from build123d import *

# Parameters (mm, degrees)
EXTRUDE_1_DEPTH     = 40
SKETCH_2_R          = 2.1
CUT_EXTRUDE_1_DEPTH = 3
SKETCH_3_R          = 11.1
SKETCH_3_R_2        = 1.6
CUT_EXTRUDE_2_DEPTH = 3
FILLET_1_R          = 3
FILLET_2_R          = 12
FILLET_3_R          = 1
FILLET_4_R          = 1


with BuildPart() as part:
    # 草图1 → 凸台-拉伸1 (new body)
    with BuildSketch(Plane.XY):
        Polygon((0, 3), (0, 0), (38.5, 0), (41.5, 0), (41.5, 3), (41.5, 42), (38.5, 42), (38.5, 3), align=None)
    extrude(amount=EXTRUDE_1_DEPTH)

    # 草图2 → 切除-拉伸1 (cut)
    with BuildSketch(Plane(origin=(41.5, 0, 0), x_dir=(0, 0, -1), z_dir=(1, 0, 0))):
        with Locations((-35, 34)):
            Circle(SKETCH_2_R)
        with Locations((-5, 34)):
            Circle(SKETCH_2_R)
        with Locations((-35, 9)):
            Circle(SKETCH_2_R)
        with Locations((-5, 9)):
            Circle(SKETCH_2_R)
    extrude(amount=-CUT_EXTRUDE_1_DEPTH, mode=Mode.SUBTRACT)

    # 草图3 → 切除-拉伸2 (cut)
    with BuildSketch(Plane.XZ):
        with Locations((18.5, 20)):
            Circle(SKETCH_3_R)
        with Locations((8.600505063, 29.899494937)):
            Circle(SKETCH_3_R_2)
        with Locations((28.399494937, 29.899494937)):
            Circle(SKETCH_3_R_2)
        with Locations((28.399494937, 10.100505063)):
            Circle(SKETCH_3_R_2)
        with Locations((8.600505063, 10.100505063)):
            Circle(SKETCH_3_R_2)
    extrude(amount=-CUT_EXTRUDE_2_DEPTH, mode=Mode.SUBTRACT)

    # 圆角1
    fillet_1_edges = [part.edges().sort_by_distance(p)[0] for p in [
        (41.5, 0, 20),
    ]]
    fillet(fillet_1_edges, radius=FILLET_1_R)

    # 圆角2
    fillet_2_edges = [part.edges().sort_by_distance(p)[0] for p in [
        (0, 1.5, 40),
        (0, 1.5, 0),
    ]]
    fillet(fillet_2_edges, radius=FILLET_2_R)

    # 圆角3
    fillet_3_edges = [part.edges().sort_by_distance(p)[0] for p in [
        (40, 42, 40),
        (40, 42, 0),
    ]]
    fillet(fillet_3_edges, radius=FILLET_3_R)

    # 圆角4
    fillet_4_edges = [part.edges().sort_by_distance(p)[0] for p in [
        (38.5, 3, 20),
    ]]
    fillet(fillet_4_edges, radius=FILLET_4_R)


solid = part.part
Part model, mm, in its own coordinate system. A direction names the side the tool comes from. Coordinates: 2 decimals unless noted, no trailing zeros. Order: outer loops, then holes, each group sorted by start corner. A loop starts at its lowest first (then second) coordinate and runs counter-clockwise, first axis right, second up. Notation, with made-up numbers: (39, -27) - (50, -27) arc R28 cw to (50, -9) - close; hole circle Ø8 at (58.25, 2). An arc over 180 degrees is marked (long way). Use CSV: the item, a comma, the result in double quotes.
Item 1: Probe probe 1 along Y at (x, z) = (40.5, 6); probe 2 along Y at (x, z) = (6.5, 26.5); probe 3 along X at (y, z) = (22, 27). List the from-to ranges inside material, lowest first.
Solved:
probe 1,"y = 0.76 to 7.15, 10.85 to 32.15, 35.85 to 42"
probe 2,"y = 0 to 3"
probe 3,"x = 38.5 to 41.5"
Item 2: Drop flat-ended pins along their axis: P1, Ø6.5, axis at y = 34, z = 5, coming from the +X side; P2, Ø12, axis at y = 31, z = 16, coming from the -X side; P3, Ø5, axis at x = 28.4, z = 10.1, coming from the +Y side. Give the stop position or say it passes through.
Solved:
P1,"stops at x = 41.5"
P2,"stops at x = 38.5"
P3,"stops at y = 3"
Item 3: Mould opens along X. For faces 3 (the face through (40.02, 31.95, 5.46)), 4 (the face through (40.6, 0.86, 20.28)), 5 (the face through (28.754, 1.479, 15.749)) say: +X half, -X half, draft (parallel to the pull), parting line (faces both ways), or undercut.
Solved:
face 3,"draft"
face 4,"+X half"
face 5,"undercut"
Item 4: Saw through at C-C on z = 20. Give the cut face in (x, y), and give its area (3 significant figures).
Solved:
outline,"(0, 0) - (7.4, 0) - (7.4, 3) - (0, 3) - close; (29.6, 0) - (38.5, 0) arc R3 ccw to (41.5, 3) - (41.5, 42) - (38.5, 42) - (38.5, 4) arc R1 cw to (37.5, 3) - (29.6, 3) - close"
area,"173 mm²"
Item 5: Saw through at A-A on y = 34. Give the cut face in (x, z).
Solved:
outline,"(38.5, 0) - (41.5, 0) - (41.5, 2.9) - (38.5, 2.9) - close; (38.5, 7.1) - (41.5, 7.1) - (41.5, 32.9) - (38.5, 32.9) - close; (38.5, 37.1) - (41.5, 37.1) - (41.5, 40) - (38.5, 40) - close"
Item 6: Saw through at B-B on x = 18.5. Give the cut face in (y, z), and give its area (3 significant figures).
Solved:
outline,"(0, 0) - (3, 0) - (3, 8.9) - (0, 8.9) - close; (0, 31.1) - (3, 31.1) - (3, 40) - (0, 40) - close"
area,"53.4 mm²"
Item 7: Saw through at D-D on z = 5. Give the cut face in (x, y).
Solved:
outline,"(2.25, 0) - (38.5, 0) arc R3 ccw to (41.5, 3) - (41.5, 6.9) - (38.5, 6.9) - (38.5, 4) arc R1 cw to (37.5, 3) - (2.25, 3) - close; (38.5, 11.1) - (41.5, 11.1) - (41.5, 31.9) - (38.5, 31.9) - close; (38.5, 36.1) - (41.5, 36.1) - (41.5, 42) - (38.5, 42) - close"
Item 8: 3-axis set-ups, long thin cutter, end or side, ignore diameter. For faces 1 (the face through (40.021, 11.082, 5.273)), 2 (the face through (32, 3, 20)): which of +Z, -Z, +X, -X, +Y, -Y reach the whole face in a straight line?
Solved:
face 1,"+X, -X"
face 2,"+Z, -Z, -X, +Y"
